Input: part model. Units: mm. Frame: model coordinates. A direction names the side the tool comes from. Give positions to 0.01 mm unless a question says otherwise; leave off trailing zeros. Loops run counter-clockwise (first coordinate to the right, second up) from the corner with the lowest first, then second, coordinate; pieces in that order, holes last. Notation, with made-up numbers: (81.5, 75) -> (118.5, 75) arc R21 ccw to (118.5, 107) -> close; hole circle Ø11 at (77.25, 27.5). An arc over 180 degrees is marked (long way). Answer in a Markdown table with one row per item. Add a question column.
```python
from build123d import *

# Parameters (mm, degrees)
F1_DEPTH = 3


with BuildPart() as f1:
    # F0 (on Front) → F1 (new body)
    with BuildSketch(Plane.XZ):
        with BuildLine():
            Line((65, 74.578316), (0, 74.578316))
            Line((0, 74.578316), (-27.7442, 74.578316))
            Line((-27.7442, 74.578316), (-20.87088, 68.810916))
            Line((-20.87088, 68.810916), (-22.734964, 66.589387))
            Line((-22.734964, 66.589387), (-30, 72.685476))
            Line((-30, 72.685476), (-30, 44.578316))
            Line((-30, 44.578316), (-30, -20.421684))
            ThreePointArc((-30, -20.421684), (-28.535534, -23.957218), (-25, -25.421684))
            Line((-25, -25.421684), (-5, -25.421684))
            ThreePointArc((-5, -25.421684), (-1.464466, -23.957218), (0, -20.421684))
            Line((0, -20.421684), (0, 44.578316))
            Line((0, 44.578316), (65, 44.578316))
            ThreePointArc((65, 44.578316), (68.535534, 46.042782), (70, 49.578316))
            Line((70, 49.578316), (70, 69.578316))
            ThreePointArc((70, 69.578316), (68.535534, 73.11385), (65, 74.578316))
        make_face()
    extrude(amount=F1_DEPTH)


solid = f1.part
```
1) Pull-direction query (X, two-part tool) for faces 1 (the face through (19, -1, 74.578)), 2 (the face through (-26.317, -1.479, 69.595)), 3 (the face through (70, -1, 59)); classes: +X half, -X half, draft (parallel to the pull), parting line (faces both ways), or undercut.
2) Section C-C on x = 10. Output: boundary loops of the cut face in (y, z), and give its area (3 significant figures).
3) Pin query (flat end, axial travel): pin 1 (1.5 mm diameter, centred on y = -2.5, z = 4.5, fed in from +X); pin 2 (1.5 mm diameter, centred on x = 35, y = -0.5, fed in from -Z); pin 3 (12 mm diameter, centred on x = 35, z = 42, fed in from +Y). Return the tip coordinate at first contact, or that it passes through.
4) Material intervals for line 1 along X through (y, z) = (-1.5, 18); line 2 along Z through (x, y) = (55, -0.8); line 3 along X through (y, z) = (-0.9, 70), sorted ascending.
5) Section B-B on z = 28. Output: boundary loops of the cut face in (x, y), and give its area (3 significant figures).
6) Section A-A on y = -1.2. Output: boundary loops of the cut face in (x, z).
7) Reachability of faces 4 (the face through (-24.356, -1.479, 71.735)), 5 (the face through (8, -3, 48)), 6 (the face through (32, -1, 44.578)) from +Z, -Z, +X, -X, +Y, -Y: full face, straight path, thin tool, end or side. Return the list, or none.
Working result:
| question | item | result |
|---|---|---|
| 1 | face 1 | draft |
| 1 | face 2 | undercut |
| 1 | face 3 | +X half |
| 2 | outline | (-3, 44.58) -> (0, 44.58) -> (0, 74.58) -> (-3, 74.58) -> close |
| 2 | area | 90.0 mm2 |
| 3 | pin 1 | stops at x = 0 |
| 3 | pin 2 | stops at z = 44.58 |
| 3 | pin 3 | stops at y = 0 |
| 4 | line 1 | x = -30 to 0 |
| 4 | line 2 | z = 44.58 to 74.58 |
| 4 | line 3 | x = -30 to -26.8, -22.29 to 69.98 |
| 5 | outline | (-30, -3) -> (0, -3) -> (0, 0) -> (-30, 0) -> close |
| 5 | area | 90.0 mm2 |
| 6 | outline | (-30, -20.42) arc R5 ccw to (-25, -25.42) -> (-5, -25.42) arc R5 ccw to (0, -20.42) -> (0, 44.58) -> (65, 44.58) arc R5 ccw to (70, 49.58) -> (70, 69.58) arc R5 ccw to (65, 74.58) -> (-27.74, 74.58) -> (-20.87, 68.81) -> (-22.73, 66.59) -> (-30, 72.69) -> close |
| 7 | face 4 | +Y, -Y |
| 7 | face 5 | +Z, -Z, +X, -X, -Y |
| 7 | face 6 | -Z, +X, +Y, -Y |
